```python
from build123d import *

# Parameters (mm, degrees)
SKETCH1_R           = 3.25
BOSS_EXTRUDE2_DEPTH = 50
SKETCH1_5_W         = 50
SKETCH1_5_H         = 50
SKETCH1_5_R         = 3.25
BOSS_EXTRUDE3_DEPTH = 10


with BuildPart() as part:
    # Sketch1 → Boss-Extrude2 (new body)
    with BuildSketch(Plane(origin=(0, 0, 0), x_dir=(1, 0, 0), z_dir=(0, 1, 0))):
        with Locations(Location((-25, 25, 0), (0, 0, 270))):
            Circle(SKETCH1_R)
    extrude(amount=BOSS_EXTRUDE2_DEPTH)

    # Sketch1_5 → Boss-Extrude3 (add)
    with BuildSketch(Plane(origin=(0, 0, 0), x_dir=(1, 0, 0), z_dir=(0, 1, 0))):
        with Locations((-25, 25)):
            Rectangle(SKETCH1_5_W, SKETCH1_5_H)
        with Locations(Location((-25, 25, 0), (0, 0, 270))):
            Circle(SKETCH1_5_R, mode=Mode.SUBTRACT)
    extrude(amount=BOSS_EXTRUDE3_DEPTH)


solid = part.part
```
For this review, take the finished solid that the model builds, in its own axes (mm). Round coordinates to 2 decimals unless told otherwise and drop trailing zeros. Loops run counter-clockwise (first coordinate to the right, second up) from the corner with the lowest first, then second, coordinate; pieces in that order, holes last.
(1) Mouldability with a two-part tool opening along X and no side actions: class faces 1 (the flat face through (-50, 5, -25)), 2 (the flat face through (-25, 10, -31)), 3 (the cylindrical face through (-26.978, 29.72, -27.579)) as released by +X, released by -X, zero draft, split by the parting line, or undercut.
Returned:
face 1: released by -X
face 2: zero draft
face 3: split by the parting line
(2) We need section B-B (x = -25). Give the boundary of the cut face in (y, z).
Returned:
outline: (0, -50) - (10, -50) - (10, -28.25) - (50, -28.25) - (50, -21.75) - (10, -21.75) - (10, 0) - (0, 0) - close
(3) We need section C-C (y = 17). Give the boundary of the cut face in (x, z).
Returned:
outline: circle Ø6.5 at (-25, -25)
(4) We need section A-A (z = -25). Give the boundary of the cut face in (x, y).
Returned:
outline: (-50, 0) - (0, 0) - (0, 10) - (-21.75, 10) - (-21.75, 50) - (-28.25, 50) - (-28.25, 10) - (-50, 10) - close
(5) We need section D-D (z = -43). Give the boundary of the cut face in (x, y), plus the area to 3 significant figures.
Returned:
outline: (-50, 0) - (0, 0) - (0, 10) - (-50, 10) - close
area: 500 mm2
(6) Clearance check with flat-ended pins moving along their axes: P1, Ø1.5, axis at x = -9, z = -42.5, coming from the +Y side; P2, Ø10, axis at x = -34, y = 33.5, coming from the -Z side. State where each tip first meets the part, or that it passes through.
Returned:
P1: stops at y = 10
P2: passes through
(7) Wall thickness on line 1 along Y through (x, z) = (-16, -7); line 2 along Z through (x, y) = (-22, 47.5); line 3 along X through (y, z) = (39, -24.5): over which ranges is each line inside the solid? List them lowest first.
Returned:
line 1: y = 0 to 10
line 2: z = -26.25 to -23.75
line 3: x = -28.21 to -21.79
